Input: dimensioned drawing with shaded views. Units: mm. Origin: part minimum x, y, z. Round coordinates to 2 decimals unless told otherwise and drop trailing zeros. Loops run counter-clockwise (first coordinate to the right, second up) from the corner with the lowest first, then second, coordinate; pieces in that order, holes last. Notation, with made-up numbers: (-31, -32) - (-25, -32) arc R10 ccw to (-25, -26) - close; hole circle Ø3 at (68, 52). An arc over 180 degrees is marked (long way). Answer as CSV lines item,"result".
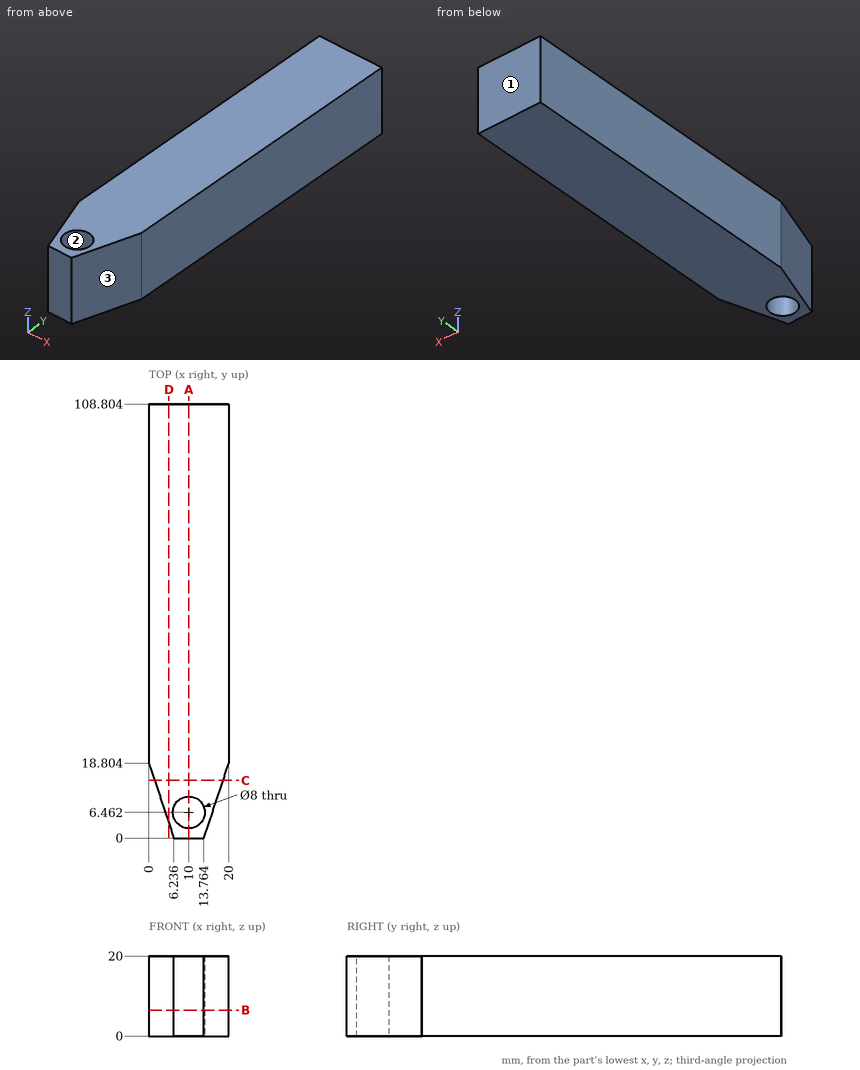
(1) Pin query (flat end, axial travel): P1, Ø6.5, axis at x = 10, y = 6.46, coming from the +Z side. Return the tip coordinate at first contact, or that it passes through.
Findings below:
P1,"through"
(2) Section C-C (y = 14.5). Output: boundary loops of the cut face in (x, z).
Findings below:
outline,"(1.43, 0) - (18.57, 0) - (18.57, 20) - (1.43, 20) - close"
(3) Section A-A (x = 10). Output: boundary loops of the cut face in (y, z) (1 decimal).
Findings below:
outline,"(0, 0) - (2.5, 0) - (2.5, 20) - (0, 20) - close; (10.5, 0) - (108.8, 0) - (108.8, 20) - (10.5, 20) - close"
(4) Section B-B (z = 6.5). Output: boundary loops of the cut face in (x, y) (1 decimal).
Findings below:
outline,"(0, 18.8) - (6.2, 0) - (13.8, 0) - (20, 18.8) - (20, 108.8) - (0, 108.8) - close; hole circle Ø8 at (10, 6.5)"
(5) Draft query along Y for the marked faces 1, 2 and 3. Return one class per face: pulls with the +Y half, pulls with the -Y half, needs draft (parallel to the pull), parting line crosses it, or undercut.
Findings below:
face 1,"pulls with the +Y half"
face 2,"undercut"
face 3,"pulls with the -Y half"
(6) Section D-D (x = 5). Output: boundary loops of the cut face in (y, z) (1 decimal), and give its area (3 significant figures).
Findings below:
outline,"(3.7, 0) - (108.8, 0) - (108.8, 20) - (3.7, 20) - close"
area,"2,100 mm2"
(7) Material intervals for line 1 along Y through (x, z) = (10, 13.5) (1 decimal); line 2 along Y through (x, z) = (7.5, 6.25) (1 decimal); line 3 along X through (y, z) = (9, 7.25), sorted ascending.
Findings below:
line 1,"0 to 2.5, 10.5 to 108.8"
line 2,"0 to 3.3, 9.6 to 108.8"
line 3,"3.25 to 6.91, 13.09 to 16.75"
